```python
from build123d import *

# Parameters (mm, degrees)
SKETCH_1_R          = 12.5
EXTRUDE_1_DEPTH     = 3
SKETCH_2_R          = 1.5
CUT_EXTRUDE_1_DEPTH = 3
SKETCH_3_R          = 2
EXTRUDE_2_DEPTH     = 20


with BuildPart() as part:
    # 草图1 → 凸台-拉伸1 (new body)
    with BuildSketch(Plane.XY):
        Circle(SKETCH_1_R)
    extrude(amount=EXTRUDE_1_DEPTH)

    # 草图2 → 切除-拉伸1 (cut)
    with BuildSketch(Plane(origin=(0, 0, 0), x_dir=(-1, 0, 0), z_dir=(0, 0, -1))):
        with Locations((0, 8.5)):
            Circle(SKETCH_2_R)
        with Locations((0, -8.5)):
            Circle(SKETCH_2_R)
    extrude(amount=-CUT_EXTRUDE_1_DEPTH, mode=Mode.SUBTRACT)

    # 草图3 → 凸台-拉伸2 (add)
    with BuildSketch(Plane(origin=(0, 0, 0), x_dir=(-1, 0, 0), z_dir=(0, 0, -1))):
        with Locations(Location((0, 0, 0), (0, 0, 180))):
            Circle(SKETCH_3_R)
    extrude(amount=EXTRUDE_2_DEPTH)


solid = part.part
```
Geometry check sheet. Reference: the model listing, model coordinates, mm. Round coordinates to 2 decimals unless told otherwise and drop trailing zeros. Loops run counter-clockwise (first coordinate to the right, second up) from the corner with the lowest first, then second, coordinate; pieces in that order, holes last. Notation, with made-up numbers: (-33.75, 57) - (-10.75, 57) arc R18 ccw to (-10.75, 90) - close; hole circle Ø5 at (5.5, -20.75). An arc over 180 degrees is marked (long way). Write each question's results on one line, items separated by ' | '. Start each with the question number.
Q1. Cross-section at D-D on z = 1.5. Enter the section's corners in (x, y).
Q2. Cross-section at A-A on x = 0. Enter the section's corners in (y, z), and give its area (3 significant figures).
Q3. Cross-section at C-C on y = 0. Enter the section's corners in (x, z), and give its area (3 significant figures).
Q4. Release check for a two-part mould opening along Y. For faces 1 (the cylindrical face through (0, 2, -10)), 2 (the flat face through (0, 0, 3)), 3 (the cylindrical face through (0, 7, 1)) record: +Y half, -Y half, draft (parallel to the pull), parting line (faces both ways), or undercut.
Q5. Thickness scan on line 1 (Y direction, x = 0, z = 2.3); line 2 (Z direction, x = 5, y = -4.5); line 3 (Y direction, x = 5.75, z = 0.75). Record the ranges inside material, lowest first. Write a range as [from, to].
Q6. Gauge pin test, flat ends, axial feed: P1, Ø1.5, axis at x = -8.5, z = -1.5, coming from the +Y side; P2, Ø8, axis at y = -1, z = -14.5, coming from the +X side; P3, Ø3.5, axis at x = 0, y = 8.5, coming from the +Z side; P4, Ø4, axis at y = 3, z = -13, coming from the -X side. Record the tip position at first contact, or that the pin passes through.
Q7. Cross-section at B-B on y = -9.5. Enter the section's corners in (x, z).
Answers below:
1) outline: circle Ø25 at (0, 0); hole circle Ø3 at (0, -8.5); hole circle Ø3 at (0, 8.5)
2) outline: (-12.5, 0) - (-10, 0) - (-10, 3) - (-12.5, 3) - close; (-7, 0) - (-2, 0) - (-2, -20) - (2, -20) - (2, 0) - (7, 0) - (7, 3) - (-7, 3) - close; (10, 0) - (12.5, 0) - (12.5, 3) - (10, 3) - close | area: 137 mm²
3) outline: (-12.5, 0) - (-2, 0) - (-2, -20) - (2, -20) - (2, 0) - (12.5, 0) - (12.5, 3) - (-12.5, 3) - close | area: 155 mm²
4) face 1: parting line | face 2: draft | face 3: undercut
5) line 1: y = [-12.5, -10], [-7, 7], [10, 12.5] | line 2: z = [0, 3] | line 3: y = [-11.1, 11.1]
6) P1: passes through | P2: stops at x = 2 | P3: stops at z = 3 | P4: stops at x = -1.73
7) outline: (-8.12, 0) - (-1.12, 0) - (-1.12, 3) - (-8.12, 3) - close; (1.12, 0) - (8.12, 0) - (8.12, 3) - (1.12, 3) - close
